Print and shaded views of the part. All mm, measured from the part's lowest x, y and z. A direction names the side the tool comes from. Round coordinates to 2 decimals unless told otherwise and drop trailing zeros. Loops run counter-clockwise (first coordinate to the right, second up) from the corner with the lowest first, then second, coordinate; pieces in that order, holes last. Notation, with made-up numbers: (15, 59) -> (28, 59) arc R5 ccw to (28, 64) -> close; hole circle Ø2 at (11, -11.75). An arc over 180 degrees is marked (long way). Answer as CSV lines item,"result".
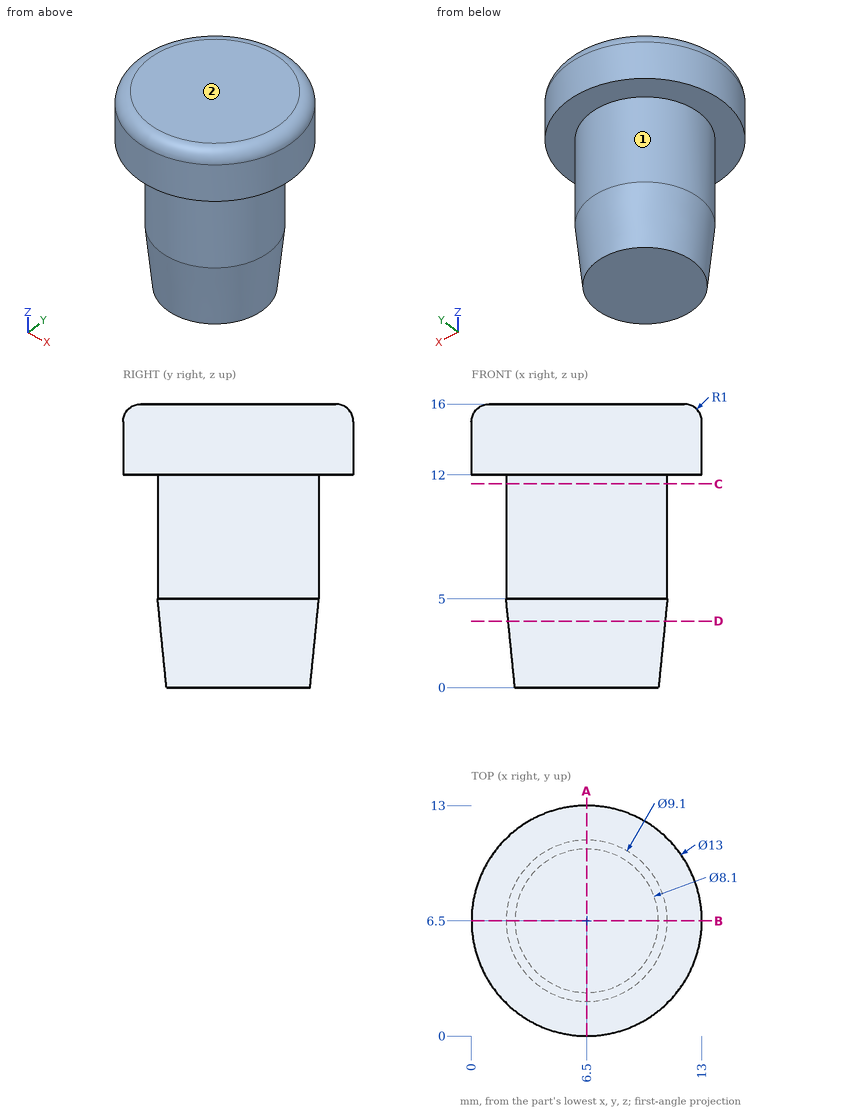
Q1. Saw through at C-C, the plane z = 11.5. Write the cut outline in (x, y), then the cut area to 3 significant figures.
Geometry results:
outline,"circle Ø9.1 at (6.5, 6.5)"
area,"65.0 mm2"
Q2. Saw through at D-D, the plane z = 3.75. Write the cut outline in (x, y) (3 decimals).
Geometry results:
outline,"circle Ø8.85 at (6.5, 6.5)"
Q3. Drop flat-ended pins along their axis: P1, Ø5, axis at y = 4, z = 10.5, coming from the +X side; P2, Ø2, axis at x = 10, z = 4, coming from the -Y side; P3, Ø1, axis at y = 7, z = 9, coming from the -X side. Give the stop position or say it passes through.
Geometry results:
P1,"x = 12.98"
P2,"y = 2.81"
P3,"x = 1.95"
Q4. Which spindle directions (+Z, -Z, +X, -X, +Y, -Y) get a long thin tool onto all of the face, cutting with end or side? Do the marked faces 1 and 2. Say none if no direction does.
Geometry results:
face 1,"-Z"
face 2,"+Z, +X, -X, +Y, -Y"
Q5. Saw through at A-A, the plane x = 6.5. Write the cut outline in (y, z), then the cut area to 3 significant figures.
Geometry results:
outline,"(0, 12) -> (1.95, 12) -> (1.95, 5) -> (2.45, 0) -> (10.55, 0) -> (11.05, 5) -> (11.05, 12) -> (13, 12) -> (13, 15) arc R1 ccw to (12, 16) -> (1, 16) arc R1 ccw to (0, 15) -> close"
area,"158 mm2"
Q6. Drill centre lines: line 1 along Z through (x, y) = (7.5, 1.25); line 2 along Y through (x, z) = (4, 13.75); line 3 along Y through (x, z) = (12.5, 15). Where is each one in solid material? Low to high.
Geometry results:
line 1,"12 to 16"
line 2,"0.5 to 12.5"
line 3,"4 to 9"
